For this review, take the finished solid that the model builds, in its own axes (mm). A direction names the side the tool comes from. Give positions to 0.01 mm unless a question says otherwise; leave off trailing zeros. Write each loop counter-clockwise with the first axis right and the second up, starting at its lowest first coordinate (ties: lowest second). Pieces come first, ordered by that corner, then holes.
from build123d import *

# Parameters (mm, degrees)
F0_W     = 12.7
F0_H     = 76.2
F1_DEPTH = 114.3
F3_DEPTH = 12.7
F4_W     = 228.6
F4_H     = 6.35
F5_DEPTH = 4.7625
F8_DEPTH = 215.9


with BuildPart() as f1:
    # F0 (on Front) → F1 (new body, symmetric)
    with BuildSketch(Plane.XZ):
        Rectangle(F0_W, F0_H)
    extrude(amount=F1_DEPTH, both=True)

    # F2 (on face) → F3 (cut, through all)
    with BuildSketch(Plane.YZ.offset(6.35)):
        Polygon((-101.6, 25.4), (-114.3, 25.4), (-114.3, 15.875), (-101.6, 13.33729), align=None)
        Polygon((-114.3, -28.575), (-114.3, -38.1), (-101.6, -38.1), (-101.6, -26.03729), align=None)
        Polygon((114.3, 28.575), (114.3, 38.1), (101.6, 38.1), (101.6, 26.03729), align=None)
        Polygon((101.6, -38.1), (114.3, -38.1), (114.3, -28.575), (101.6, -26.03729), align=None)
    extrude(amount=-F3_DEPTH, mode=Mode.SUBTRACT)

    # F4 (on face) → F5 (cut)
    with BuildSketch(Plane(origin=(-6.35, 0, 0), x_dir=(0, -1, 0), z_dir=(-1, 0, 0))):
        with Locations((0, 28.575)):
            Rectangle(F4_W, F4_H)
    extrude(amount=-F5_DEPTH, mode=Mode.SUBTRACT)

    # F7 (on face) → F8 (cut, through all)
    with BuildSketch(Plane.XZ.offset(114.3)):
        with BuildLine():
            ThreePointArc((0, 34.925), (0.929936, 37.170064), (3.175, 38.1))
            Line((3.175, 38.1), (0, 38.1))
            Line((0, 38.1), (0, 34.925))
        make_face()
        with BuildLine():
            ThreePointArc((3.175, 38.1), (5.420064, 37.170064), (6.35, 34.925))
            Line((6.35, 34.925), (6.35, 38.1))
            Line((6.35, 38.1), (3.175, 38.1))
        make_face()
    extrude(amount=-F8_DEPTH, mode=Mode.SUBTRACT)


solid = f1.part
(1) The part is to be moulded in two halves that separate along Y. For faces 1 (the flat face through (0, 101.6, 32)), 2 (the flat face through (0, 114.3, 0)), 3 (the flat face through (0, -101.6, 19)), 4 (the flat face through (-6.35, -8, 35)), say which applies: +Y half, -Y half, draft (parallel to the pull), parting line (faces both ways), or undercut.
(2) We need section A-A (x = -3.5). Write out the cut boundary in (y, z) (3 decimals).
(3) For L1, parallel to Z at x = -4.5, y = 101.5; L2, parallel to Y at x = 4, z = 16; L3, parallel to Y at x = 6.25, z = -29, list the stretches that pass through material, from the lowest coordinate up.
(4) Tool access review of faces 5 (the flat face through (0.089, -108.039, 14.624)), 6 (the flat face through (-1.587, 2, 29)), 7 (the flat face through (0, 101.6, -32)), 8 (the flat face through (2.44, 107.86, 27.29)), 9 (the flat face through (2, -108, 25.4)): name each direction out of +Z, -Z, +X, -X, +Y, -Y from which nothing blocks a thin tool from reaching the whole face with its end or side.
(5) Clearance check with a flat-ended pin moving along its axis: pin 1 Ø6.5 at (x, y) = (1.5, -110) entering from -Z. State where the tip first meets the part, or that it passes through.
The answers:
1. face 1: undercut
1. face 2: +Y half
1. face 3: undercut
1. face 4: draft
2. outline: (-114.3, -28.575) - (-101.6, -26.037) - (-101.6, -38.1) - (101.6, -38.1) - (101.6, -26.037) - (114.3, -28.575) - (114.3, 25.4) - (-101.6, 25.4) - (-101.6, 13.337) - (-114.3, 15.875) - close; (-114.3, 31.75) - (101.6, 31.75) - (101.6, 38.1) - (-114.3, 38.1) - close
3. L1: z = -38.1 to 25.4, 31.75 to 38.1
3. L2: y = -101.6 to 114.3
3. L3: y = -101.6 to 101.6
4. face 5: +X, -X
4. face 6: -X, +Y, -Y
4. face 7: -Z, +X, -X
4. face 8: +Z, +X, -X
4. face 9: +X, -X, -Y
5. pin 1: stops at z = -28.37
